```python
from build123d import *

# Parameters (mm, degrees)
F1_DEPTH = 34.4
F2_W     = 83.3284929395
F2_H     = 77.8343044221
F3_DEPTH = 24.3
F5_DEPTH = 25
F7_DEPTH = 25


with BuildPart() as f1:
    # F0 (on Top) → F1 (new body, symmetric)
    with BuildSketch(Plane.XY):
        Polygon((50.8212260902, 18.5428783298), (50.8212260902, 59.2914260924), (-50.8212260902, 59.2914260924), (-50.8212260902, -59.2914260924), (-32.5072668493, -59.2914260924), (-32.5072668493, 18.5428783298), align=None)
    extrude(amount=F1_DEPTH, both=True)

    # F2 (on face) → F3 (join)
    with BuildSketch(Plane(origin=(0, 0, -34.4), x_dir=(1, 0, 0), z_dir=(0, 0, -1))):
        with Locations((9.1569796205, 20.3742738813)):
            Rectangle(F2_W, F2_H)
    extrude(amount=-F3_DEPTH)

    # F4 (on face) → F5 (join)
    with BuildSketch(Plane.YZ.offset(-32.5072668493)):
        Polygon((18.5428783298, 34.4), (-59.2914260924, -10.1), (18.5428783298, -10.1), align=None)
    extrude(amount=F5_DEPTH)

    # F6 (on face) → F7 (cut)
    with BuildSketch(Plane.XZ.offset(59.2914260924)):
        Polygon((50.8212260902, -10.1), (-7.5072668493, -10.1), (28.6875050515, -21.577918902), (28.6875050515, -34.4), (50.8212260902, -34.4), align=None)
    extrude(amount=-F7_DEPTH, mode=Mode.SUBTRACT)


solid = f1.part
```
Geometry check sheet. Reference: the model listing, model coordinates, mm. A direction names the side the tool comes from. Round coordinates to 2 decimals unless told otherwise and drop trailing zeros. Order: outer loops, then holes, each group sorted by start corner. A loop starts at its lowest first (then second) coordinate and runs counter-clockwise, first axis right, second up. Notation, with made-up numbers: (50.25, 60.25) - (72.25, 60.25) arc R22 ccw to (72.25, 73.25) - close; hole circle Ø9 at (-12.5, 45). An arc over 180 degrees is marked (long way). Use a Markdown table: item, result. Add a question column.
(1) Tool access check on faces 1 (the flat face through (28.688, -47, -28)), 2 (the flat face through (-32.507, -30, 17)), 3 (the flat face through (-12, 27, 34.4)). Record the directions out of +Z, -Z, +X, -X, +Y, -Y that give a thin tool (end or side, any length) a straight path to the whole face; none if there is none.
(2) Sectioned sample at D-D, the plane z = -26. Enter the section's corners in (x, y).
(3) Material ranges on line 1 along Y through (x, z) = (30.5, 15.5); line 2 along Y through (x, z) = (30.5, -10.5); line 3 along Z through (x, y) = (3, -14), recorded low to high. Write a range as [from, to].
(4) Sectioned sample at B-B, the plane z = 24.5. Enter the section's corners in (x, y), and give its area (3 significant figures).
(5) Depth check by flat-ended pin: pin 1 (13.5 mm diameter, centred on x = 10, z = 5, fed in from -Y); pin 2 (12 mm diameter, centred on y = -28, z = 18, fed in from +X); pin 3 (13.5 mm diameter, centred on y = -14, z = 23, fed in from +X). Enter the tip coordinate at first touch or a pass-through.
(6) Sectioned sample at A-A, the plane x = -16.5. Enter the section's corners in (y, z).
(7) Sectioned sample at C-C, the plane y = 6. Enter the section's corners in (x, z).
(8) Release check for a two-part mould opening along Y. For faces 4 (the flat face through (-20, -59.291, -16)), 5 (the flat face through (1, 59.291, 0)), 6 (the flat face through (-1, -1, -34.4)) record: pulls with the +Y half, pulls with the -Y half, needs draft (parallel to the pull), parting line crosses it, or undercut.
Answers below:
| question | item | result |
|---|---|---|
| 1 | face 1 | +Z, -Z, +X, -Y |
| 1 | face 2 | +Z, +X, -Y |
| 1 | face 3 | +Z, +X, -X, +Y, -Y |
| 2 | outline | (-50.82, -59.29) - (28.69, -59.29) - (28.69, -34.29) - (50.82, -34.29) - (50.82, 59.29) - (-50.82, 59.29) - close |
| 3 | line 1 | [18.54, 59.29] |
| 3 | line 2 | [-34.29, 59.29] |
| 3 | line 3 | [-34.4, -10.1] |
| 4 | outline | (-50.82, -59.29) - (-32.51, -59.29) - (-32.51, 1.23) - (-7.51, 1.23) - (-7.51, 18.54) - (50.82, 18.54) - (50.82, 59.29) - (-50.82, 59.29) - close |
| 4 | area | 6,000 mm² |
| 5 | pin 1 | y = 18.54 |
| 5 | pin 2 | x = -32.51 |
| 5 | pin 3 | x = -7.51 |
| 6 | outline | (-59.29, -34.4) - (59.29, -34.4) - (59.29, 34.4) - (18.54, 34.4) - (-59.29, -10.1) - close |
| 7 | outline | (-50.82, -34.4) - (50.82, -34.4) - (50.82, -10.1) - (-7.51, -10.1) - (-7.51, 27.23) - (-32.51, 27.23) - (-32.51, 34.4) - (-50.82, 34.4) - close |
| 8 | face 4 | pulls with the -Y half |
| 8 | face 5 | pulls with the +Y half |
| 8 | face 6 | needs draft |
